Build history of the part. All positions in model axes, mm. Face numbers are marked on the shaded views. A direction names the side the tool comes from. Give positions to 0.01 mm unless a question says otherwise; leave off trailing zeros. Loops run counter-clockwise (first coordinate to the right, second up) from the corner with the lowest first, then second, coordinate; pieces in that order, holes last. Notation, with made-up numbers: (-25.5, 44.25) -> (17.5, 44.25) arc R24 ccw to (17.5, 79.25) -> close; hole circle Ø3 at (30.5, -40). An arc over 180 degrees is marked (long way). One line per question, with ' | ' between items. Start each with the question number.
(1) Slice it at D-D, the plane y = -5.5. Write the cut outline in (x, z), then the cut area to 3 significant figures.
(2) Mould opens along Y. For the marked faces 4, 5, 6 and 7 say: pulls with the +Y half, pulls with the -Y half, needs draft (parallel to the pull), parting line crosses it, or undercut.
(3) 3-axis set-ups, long thin cutter, end or side, ignore diameter. For the marked faces 1, 2 and 3: which of +Z, -Z, +X, -X, +Y, -Y reach the whole face in a straight line?
(4) Slice it at B-B, the plane x = 0. Write the cut outline in (y, z).
(5) Drill centre lines: L1, parallel to Y at x = 55, z = 22; L2, parallel to Y at x = 55, z = 8; L3, parallel to Y at x = 0, z = 63. Where is each one in solid material? Low to high. Write a range as from..to.
(6) Flat gauge pins, fed straight in: pin 1 Ø12 at (x, z) = (-33, 17) entering from +Y; pin 2 Ø5 at (y, z) = (22, 40) entering from -X; pin 3 Ø2 at (x, z) = (-12.5, 61.5) entering from -Y; pin 4 Ø24 at (x, y) = (55, 5) entering from -Z. Where does each tip first touch, or does it go through?
(7) Slice it at C-C, the plane y = 8.5. Write the cut outline in (x, z), then the cut area to 3 significant figures.
(8) Slice it at A-A, the plane z = 18. Write the cut outline in (x, y).
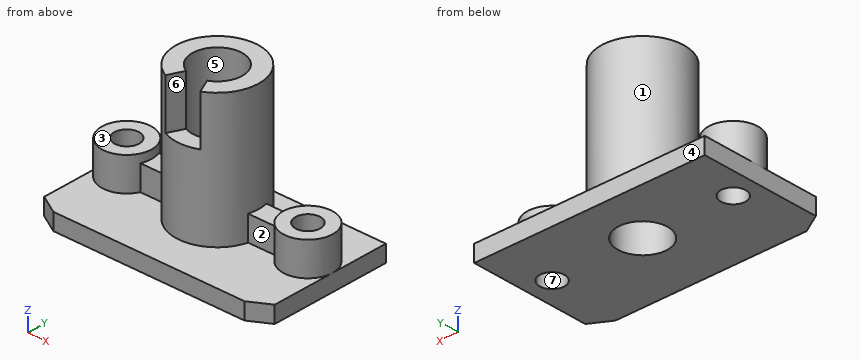
```python
from build123d import *

# Parameters (mm, degrees)
SKETCH_W        = 140
SKETCH_H        = 80
SKETCH_R        = 7.5
SKETCH_R_2      = 15
PAD_DEPTH       = 10
POCKET_DEPTH    = 11
SKETCH004_R     = 25
SKETCH004_R_2   = 15
PAD001_DEPTH    = 80
SKETCH005_R     = 15
SKETCH005_R_2   = 7.5
PAD002_DEPTH    = 20
SKETCH006_W     = 26
SKETCH006_H     = 12
PAD003_DEPTH    = 15
POCKET001_DEPTH = 30


with BuildPart() as part:
    # Sketch → Pad (new body)
    with BuildSketch(Plane.XY):
        Rectangle(SKETCH_W, SKETCH_H)
        with Locations((-55, 5)):
            Circle(SKETCH_R, mode=Mode.SUBTRACT)
        with Locations((55, 5)):
            Circle(SKETCH_R, mode=Mode.SUBTRACT)
        with Locations((0, 5)):
            Circle(SKETCH_R_2, mode=Mode.SUBTRACT)
    extrude(amount=PAD_DEPTH)

    # Sketch001 (on Face9 of Pad) → Pocket (cut)
    with BuildSketch(Plane.XY.offset(10)):
        Polygon((-70, -33.071797), (-58, -40), (-70, -40), align=None)
        Polygon((70, -33.071797), (70, -40), (58, -40), align=None)
    extrude(amount=-POCKET_DEPTH, mode=Mode.SUBTRACT)

    # Sketch004 → Pad001 (join)
    with BuildSketch(Plane.XY.offset(10)):
        with Locations((0, 5)):
            Circle(SKETCH004_R)
        with Locations((0, 5)):
            Circle(SKETCH004_R_2, mode=Mode.SUBTRACT)
    extrude(amount=PAD001_DEPTH)

    # Sketch005 (on Face4 of Pad001) → Pad002 (join)
    with BuildSketch(Plane.XY.offset(10)):
        with Locations((55, 5)):
            Circle(SKETCH005_R)
        with Locations((55, 5)):
            Circle(SKETCH005_R_2, mode=Mode.SUBTRACT)
        with Locations((-55, 5)):
            Circle(SKETCH005_R)
        with Locations((-55, 5)):
            Circle(SKETCH005_R_2, mode=Mode.SUBTRACT)
    extrude(amount=PAD002_DEPTH)

    # Sketch006 (on Face4 of Pad002) → Pad003 (join)
    with BuildSketch(Plane.XY.offset(10)):
        with Locations((-33.01482, 5)):
            Rectangle(SKETCH006_W, SKETCH006_H)
        with Locations((33.01482, 5)):
            Rectangle(SKETCH006_W, SKETCH006_H)
    extrude(amount=PAD003_DEPTH)

    # Sketch007 (on Face21 of Pad003) → Pocket001 (cut)
    with BuildSketch(Plane.XY.offset(90)):
        with BuildLine():
            ThreePointArc((-10.565449, -17.657698), (1e-06, -20), (10.56545, -17.657698))
            Line((10.56545, -17.657698), (0, 5))
            Line((0, 5), (-10.565449, -17.657698))
        make_face()
    extrude(amount=-POCKET001_DEPTH, mode=Mode.SUBTRACT)


solid = part.part
```
Final values:
1) outline: (-70, 0) -> (-10.71, 0) -> (-10.71, 90) -> (-22.69, 90) -> (-22.69, 10) -> (-44.29, 10) -> (-44.29, 30) -> (-65.71, 30) -> (-65.71, 10) -> (-70, 10) -> close; (10.71, 0) -> (70, 0) -> (70, 10) -> (65.71, 10) -> (65.71, 30) -> (44.29, 30) -> (44.29, 10) -> (22.69, 10) -> (22.69, 90) -> (10.71, 90) -> close | area: 3,960 mm2
2) face 4: pulls with the +Y half | face 5: undercut | face 6: pulls with the -Y half | face 7: undercut
3) face 1: +Z | face 2: +Z, -Y | face 3: +Z, -X, +Y, -Y
4) outline: (-40, 0) -> (-10, 0) -> (-10, 60) -> (-20, 60) -> (-20, 10) -> (-40, 10) -> close; (20, 0) -> (40, 0) -> (40, 10) -> (30, 10) -> (30, 90) -> (20, 90) -> close
5) L1: -10..-2.5, 12.5..20 | L2: -40..-2.5, 12.5..40 | L3: 20..30
6) pin 1: y = 11 | pin 2: x = -20.37 | pin 3: y = -17.2 | pin 4: z = 0
7) outline: (-70, 0) -> (-61.63, 0) -> (-61.63, 30) -> (-69.59, 30) -> (-69.59, 10) -> (-70, 10) -> close; (-48.37, 0) -> (-14.59, 0) -> (-14.59, 90) -> (-24.75, 90) -> (-24.75, 25) -> (-40.41, 25) -> (-40.41, 30) -> (-48.37, 30) -> close; (14.59, 0) -> (48.37, 0) -> (48.37, 30) -> (40.41, 30) -> (40.41, 25) -> (24.75, 25) -> (24.75, 90) -> (14.59, 90) -> close; (61.63, 0) -> (70, 0) -> (70, 10) -> (69.59, 10) -> (69.59, 30) -> (61.63, 30) -> close | area: 3,580 mm2
8) outline: (-41.25, -1) -> (-24.27, -1) arc R25 ccw to (24.27, -1) -> (41.25, -1) arc R15 ccw (long way) to (41.25, 11) -> (24.27, 11) arc R25 ccw to (-24.27, 11) -> (-41.25, 11) arc R15 ccw (long way) to start; hole circle Ø15 at (-55, 5); hole circle Ø30 at (0, 5); hole circle Ø15 at (55, 5)
